Check sheet for the modelled part. Datum: model origin and axes. Units: mm. A direction names the side the tool comes from. Give positions to 0.01 mm unless a question says otherwise; leave off trailing zeros. Write each loop counter-clockwise with the first axis right and the second up, starting at its lowest first coordinate (ties: lowest second). Pieces come first, ordered by that corner, then holes. Notation, with made-up numbers: (37.25, 5.5) - (86.25, 5.5) arc R17 cw to (86.25, 26.5) - close; hole circle Ø11 at (-17.75, -1.5). An arc over 180 degrees is marked (long way). Return JSON: item names as keys, results as strings. Group by question number.
Autodesk Inventor part; units mm, degrees
ref_plane "YZ Plane" through (0, 0, 0) normal (1, 0, 0) x (0, 1, 0)
ref_plane "XZ Plane" through (0, 0, 0) normal (0, 1, 0) x (-1, 0, 0)
ref_plane "XY Plane" through (0, 0, 0) normal (0, 0, 1) x (1, 0, 0)
ref_plane "Work Plane1" through (-37.0541, 3.9333, 19.6842) normal (0, 1, 0) x (-1, 0, 0)
sketch "Sketch1" plane through (-37.0541, 3.9333, 19.6842) normal (0, 1, 0) x (-1, 0, 0)
  point P0 (-37.0541, -19.6842)
ref_plane "Work Plane2" through (-37.0541, 26.9333, 19.6842) normal (0, 1, 0) x (-1, 0, 0)
sketch "Sketch2" plane through (-37.0541, 26.9333, 19.6842) normal (0, 1, 0) x (-1, 0, 0)
  line L0 (-16.9, -6.2922) -> (-16.9, -34.5181) construction
  line L1 (-18.4, -45.1) -> (-15.4, -45.1)
  line L2 (-15.4, 4.9) -> (-18.4, 4.9)
  line L3 (-15.4, -45.1) -> (-16.9, -20.1) construction
  line L4 (-17.065, -17.35) -> (-18.4, 4.9) construction
  line L5 (26.6, -17.35) -> (-15.4, -17.35)
  line L6 (-16.735, -17.35) -> (-17.065, -17.35)
  line L7 (-18.4, -17.35) -> (-60.4, -17.35)
  line L8 (-18.4, 4.9) -> (-18.4, -17.35)
  line L9 (-18.4, -22.85) -> (-18.4, -45.1)
  line L10 (-15.4, -45.1) -> (-15.4, -22.85)
  line L11 (-15.4, -17.35) -> (-15.4, 4.9)
  line L12 (-15.4, -22.85) -> (26.6, -22.85)
  line L13 (-18.4, -45.1) -> (-17.065, -22.85) construction
  line L14 (-16.9, -20.1) -> (-15.4, 4.9) construction
  line L15 (-60.4, -22.85) -> (-18.4, -22.85)
  line L16 (-17.065, -22.85) -> (-16.735, -22.85)
  line L17 (-60.4, -17.35) -> (-60.4, -22.85)
  line L18 (26.6, -17.35) -> (26.6, -22.85)
  point P0 (-37.0541, -19.6842)
  point P1 (22.6, -17.35)
  point P2 (-56.4, -22.85)
  dimension "d3" = 3
  dimension "d4" = 50
  dimension "d5" = 42
  dimension "d6" = 42
extrude "Extrusion2" add sketch "Sketch2" along normal blind 3
sketch "Sketch3" plane through (-37.0541, 26.9333, 19.6842) normal (0, -1, 0) x (1, 0, 0)
  line L0 (60.4, -22.85) -> (18.4, -22.85)
  line L1 (18.4, -17.35) -> (60.4, -17.35)
  line L2 (60.4, -22.85) -> (56.4, -22.85)
  line L3 (56.4, -22.85) -> (56.4, -17.35)
  line L4 (56.4, -17.35) -> (60.4, -17.35)
  line L5 (60.4, -17.35) -> (60.4, -22.85)
  line L6 (-26.6, -22.85) -> (-26.6, -17.35)
  line L7 (-26.6, -17.35) -> (15.4, -17.35)
  line L8 (-26.6, -22.85) -> (-22.6, -22.85)
  line L9 (-22.6, -22.85) -> (-22.6, -17.35)
  line L10 (-22.6, -17.35) -> (-26.6, -17.35)
  line L11 (-26.6, -17.35) -> (-26.6, -22.85)
  point P0 (37.0541, -19.6842)
  dimension "d9" = 4
  dimension "d10" = 4
extrude "Extrusion3" add sketch "Sketch3" along normal blind 23
sketch "Sketch4" plane through (19.3459, 26.9333, -3.1658) normal (-1, 0, 0) x (0, 0, 1)
  line L0 (5.5, -23) -> (0, -23)
  line L1 (5.5, 0) -> (5.5, -23)
  line L2 (0, -23) -> (5.5, -23)
  line L3 (5.5, -23) -> (5.5, -19)
  line L4 (5.5, -19) -> (0, -19)
  line L5 (0, -19) -> (0, -23)
  point P0 (3.1658, -26.9333)
  dimension "d13" = 4
sketch "Sketch5" plane through (-18.6541, 29.9333, 2.3342) normal (0, 0, 1) x (1, 0, 0)
  line L0 (38, -3) -> (38, -26)
  line L1 (38, -26) -> (32.5, -26)
  line L2 (32.5, -26) -> (32.5, -23)
  line L3 (32.5, -23) -> (38, -17.8732)
  point P0 (18.6541, -29.9333)
  dimension "d14" = 5.5
  dimension "d15" = 3
extrude "Extrusion4" add sketch "Sketch5" against normal up to surface (5.5 mm away)
ref_plane "Work Plane3" through (-20.1541, 26.9333, 2.3342) normal (1, 0, 0) x (0, 0, -1)
mirror "Mirror1" about plane through (-20.1541, 26.9333, 2.3342) normal (1, 0, 0) of "Extrusion4"
ref_plane "Work Plane4" through (-37.0541, 12.1833, 19.6842) normal (0, -1, 0) x (1, 0, 0)
sketch "Sketch6" plane through (-37.0541, 12.1833, 19.6842) normal (0, -1, 0) x (1, 0, 0)
  circle A0 centre (53.4, -20.1) radius 1.7
  circle A1 centre (-19.6, -20.1) radius 1.7
  line L0 (-16.8355, -21.7765) -> (-19.6696, -23.3324)
  line L1 (-19.6696, -23.3324) -> (-22.4342, -21.6559)
  line L2 (-22.4342, -21.6559) -> (-22.3645, -18.4234)
  line L3 (-22.3645, -18.4234) -> (-19.5303, -16.8676)
  line L4 (-19.5303, -16.8676) -> (-16.7658, -18.5441)
  line L5 (-16.7658, -18.5441) -> (-16.8355, -21.7765)
  line L6 (-19.6696, -23.3324) -> (-15.5487, -23.3324)
  line L7 (-15.5487, -23.3324) -> (-15.5487, -16.0828)
  line L8 (-15.5487, -16.0828) -> (-19.5303, -16.8676)
  point P0 (37.0541, -19.6842)
  dimension "d19" = 5.6
extrude "Extrusion5" cut sketch "Sketch6" along normal blind 5.25 contours A1 | L5 L4 L8 L7 L6 L0 | L0 L1 L2 L3 L4 L5
sketch "Sketch7" plane through (-37.0541, 3.9333, 19.6842) normal (0, -1, 0) x (1, 0, 0)
  circle A0 centre (-19.6, -20.1) radius 1.7
  point P0 (37.0541, -19.6842)
extrude "Extrusion6" cut sketch "Sketch7" against normal blind 6.25
mirror "Mirror2" about plane through (-20.1541, 26.9333, 2.3342) normal (1, 0, 0) of "Extrusion5", "Extrusion6"
properties part number "tec_holder_part2"
Item 1: Access from +Z, -Z, +X, -X, +Y, -Y to the whole of each face (thin tool, end or side, straight path). Record for faces 4 (the face through (18.119, 8.876, 1.805)), 5 (the face through (13.846, 5, 0)), 6 (the face through (18.044, 5.412, -0.491)), 7 (the face through (-51, 28, -3.166)), 8 (the face through (-18.654, 28, -14)).
Item 2: Section check A-A on y = 22.25. Record the cut outline in (x, z).
Item 3: Material ranges on line 1 along X through (y, z) = (23, 0); line 2 along X through (y, z) = (7.25, 1.5); line 3 along X through (y, z) = (28.5, -10.5), recorded low to high. Write a range as from..to.
Item 4: Depth check by flat-ended pin: pin 1 (15 mm diameter, centred on x = -19.5, z = 8, fed in from -Y); pin 2 (8 mm diameter, centred on x = 7.5, y = 23, fed in from +Z); pin 3 (5 mm diameter, centred on y = 11, z = 2.5, fed in from -X); pin 4 (3.5 mm diameter, centred on y = 28.5, z = 15, fed in from +X). Enter the tip coordinate at first touch or a pass-through.
Item 5: Section check B-B on x = -56.5. Record the cut outline in (y, z), plus the area to 3 significant figures.
Item 6: Section check C-C on z = -15.5. Record the cut outline in (x, y).
Item 7: Section check D-D on x = 11.5. Record the cut outline in (y, z).
Item 8: Mould release check, pull along Y, two halves, no side actions. Record for faces 1 (the face through (-58.352, 5.412, -0.341)), 2 (the face through (18, 6.933, -2)), 3 (the face through (19, 3.933, 0)): +Y half, -Y half, draft (parallel to the pull), parting line (faces both ways), or undercut.
Reply:
{
 "1": {"face 4": "none", "face 5": "+Z, -Z, -Y", "face 6": "-Y", "face 7": "-Z, -X, +Y, -Y", "face 8": "-Z, +X, +Y, -Y"},
 "2": {"outline": "(-63.65, -3.17) - (-59.65, -3.17) - (-59.65, 2.33) - (-63.65, 2.33) - close; (19.35, -3.17) - (23.35, -3.17) - (23.35, 2.33) - (19.35, 2.33) - close"},
 "3": {"line 1": "-63.65..-59.65, 19.35..23.35", "line 2": "-63.65..-58.98, 18.67..23.35", "line 3": "-21.65..-18.65"},
 "4": {"pin 1": "y = 26.93", "pin 2": "z = 2.33", "pin 3": "x = -63.65", "pin 4": "x = -18.65"},
 "5": {"outline": "(3.93, -3.17) - (6.93, -3.17) - (6.93, -2.11) - (3.93, -2.11) - close; (3.93, 1.28) - (6.93, 1.28) - (6.93, 2.33) - (3.93, 2.33) - close; (26.93, -3.17) - (29.93, -3.17) - (29.93, 2.33) - (26.93, 2.33) - close", "area": "22.8 mm²"},
 "6": {"outline": "(-21.65, 26.93) - (-18.65, 26.93) - (-18.65, 29.93) - (-21.65, 29.93) - close"},
 "7": {"outline": "(26.93, -3.17) - (29.93, -3.17) - (29.93, 2.33) - (26.93, 2.33) - close"},
 "8": {"face 1": "draft", "face 2": "undercut", "face 3": "-Y half"}
}
